Geometry: see drawing. Coordinates: mm, zero at the bounding-box minimum. Coordinates: 2 decimals unless noted, no trailing zeros. Write each loop counter-clockwise with the first axis right and the second up, starting at its lowest first coordinate (ties: lowest second). Pieces come first, ordered by that corner, then holes. Notation, with made-up numbers: M 24.5,57.25 L 67.5,57.25 A17 cw 67.5,69.25 Z; hole C 88.25,-4 d11. An arc over 180 degrees is marked long. Write item = value, one per line. Start each with the question number.
1. Section query D-D (x = 81). Output: boundary loops of the cut face in (y, z), then the cut area to 3 significant figures.
2. Line query: line 1 along X through (y, z) = (51, 64.5); line 2 along Y through (x, z) = (70, 102); line 3 along Y through (x, z) = (7, 148). Output: solid intervals per line, ascending.
3. Section query A-A (y = 100). Output: boundary loops of the cut face in (x, z).
4. Section query B-B (x = 43.5). Output: boundary loops of the cut face in (y, z).
5. Section query C-C (z = 213). Output: boundary loops of the cut face in (x, y), then the cut area to 3 significant figures.
6. Pin query (flat end, axial travel): pin 1 Ø10 at (x, y) = (41.5, 74) entering from +Z; pin 2 Ø1.5 at (x, z) = (63.5, 68.5) entering from -Y; pin 3 Ø8 at (x, y) = (73.5, 82.5) entering from +Z; pin 4 Ø8 at (x, y) = (22, 101.5) entering from -Z. Return the tip coordinate at first contact, or that it passes through.
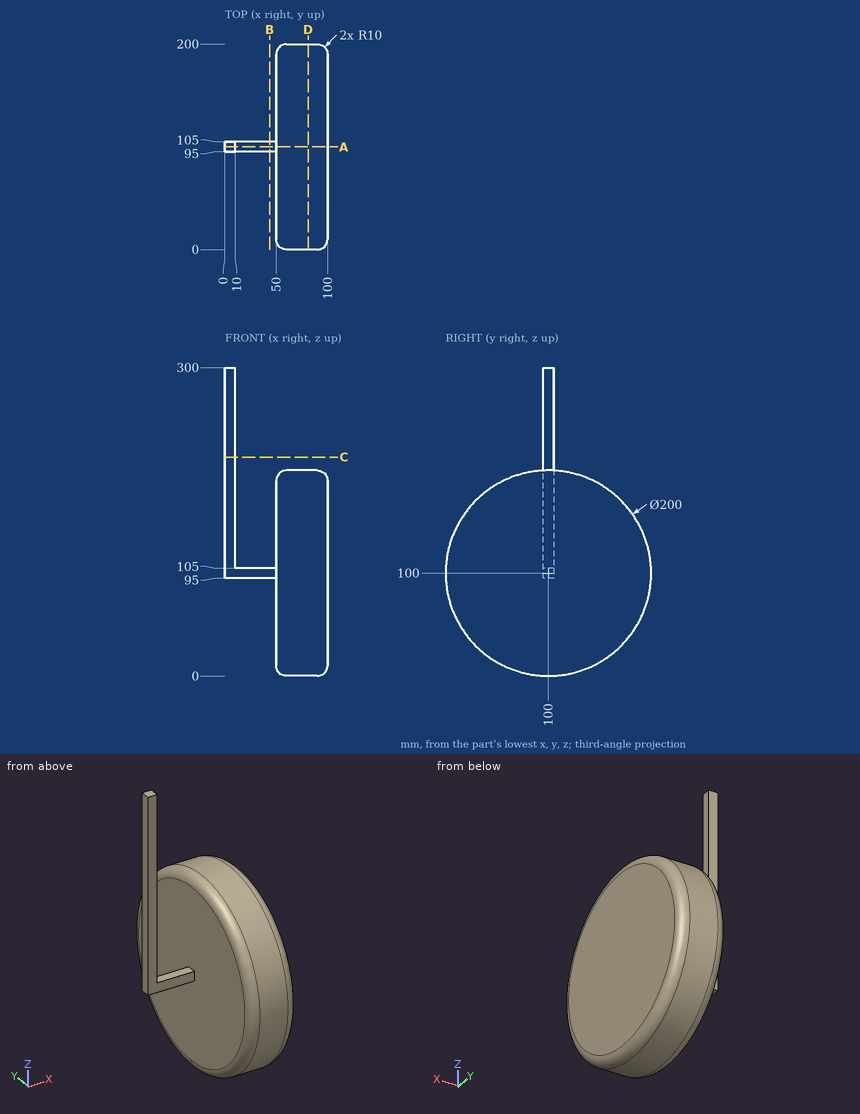
Results are:
q1.outline = C 100,100 d200
q1.area = 31,400 mm^2
q2.line_1 = 50 to 100
q2.line_2 = 0.02 to 199.98
q2.line_3 = 95 to 105
q3.outline = M 0,95 L 50,95 L 50,10 A10 ccw 60,0 L 90,0 A10 ccw 100,10 L 100,190 A10 ccw 90,200 L 60,200 A10 ccw 50,190 L 50,105 L 10,105 L 10,300 L 0,300 Z
q4.outline = M 95,95 L 105,95 L 105,105 L 95,105 Z
q5.outline = M 0,95 L 10,95 L 10,105 L 0,105 Z
q5.area = 100 mm^2
q6.pin_1 = through
q6.pin_2 = 4.85
q6.pin_3 = 199.08
q6.pin_4 = 95
